Input: part model. Units: mm. Frame: model coordinates. A direction names the side the tool comes from. Coordinates: 2 decimals unless noted, no trailing zeros. Write each loop counter-clockwise with the first axis right and the second up, starting at its lowest first coordinate (ties: lowest second). Pieces come first, ordered by that corner, then holes. Notation, with made-up numbers: M 84,42 L 124,42 A21 cw 124,80 Z; hole C 18,70 d5. An arc over 180 degrees is marked long. Write each question's results on one line, items separated by ' | '. Start each with the question number.
1. Section query A-A, the plane y = 205. Output: boundary loops of the cut face in (x, z).
2. Pull-direction query (Y, two-part tool) for faces 3 (the flat face through (203.2, 154, 3)), 4 (the cylindrical face through (173.115, 253.638, 3.131)), 5 (the cylindrical face through (201.29, 1.81, 3.22)); classes: +Y half, -Y half, draft (parallel to the pull), parting line (faces both ways), or undercut.
3. Section query B-B, the plane x = 126.5. Output: boundary loops of the cut face in (y, z), and give its area (3 significant figures).
4. First-contact query: pin 1 (4.5 mm diameter, centred on x = 190.5, y = 241.3, fed in from -Z); pin 2 (1.5 mm diameter, centred on x = 167, z = 1.5, fed in from +Y); pin 3 (3 mm diameter, centred on y = 176.5, z = 2, fed in from -X); pin 4 (1.9 mm diameter, centred on x = 101, z = 3.5, fed in from +Y). Flat tips, straight axial feed; report the tip coordinate or a pass-through.
5. Set-up query: faces 1 (the flat face through (177.8, 138, 3)), 2 (the flat face through (95, 142, 0)). Return all of +Z, -Z, +X, -X, +Y, -Y with unobstructed straight access to the full face (end or side cutting, diameter ignored); none if empty.
6. Ray query, probe 1 along Y at (x, z) = (139.7, 5); probe 2 along Y at (x, z) = (38.1, 4.25); probe 3 along X at (y, z) = (133, 0.75). Return the intervals inside material, ascending.
```python
from build123d import *

# Parameters (mm, degrees)
BOSS_EXTRUDE1_DEPTH = 6.35
SKETCH2_R           = 2.4892
CUT_EXTRUDE1_DEPTH  = 7.35
FILLET1_R           = 6.35


with BuildPart() as part:
    # Sketch1 → Boss-Extrude1 (new body)
    with BuildSketch(Plane.XY):
        Polygon((0, 25.4), (177.8, 304.8), (203.2, 304.8), (203.2, 0), (0, 0), align=None)
    extrude(amount=BOSS_EXTRUDE1_DEPTH)

    # Sketch2 → Cut-Extrude1 (cut, through all)
    with BuildSketch(Plane.XY.offset(6.35)):
        with Locations((190.5, 12.7)):
            Circle(SKETCH2_R)
        with Locations((165.1, 12.7)):
            Circle(SKETCH2_R)
        with Locations((139.7, 12.7)):
            Circle(SKETCH2_R)
        with Locations((114.3, 12.7)):
            Circle(SKETCH2_R)
        with Locations((88.9, 12.7)):
            Circle(SKETCH2_R)
        with Locations((63.5, 12.7)):
            Circle(SKETCH2_R)
        with Locations((38.1, 12.7)):
            Circle(SKETCH2_R)
        with Locations((190.5, 38.1)):
            Circle(SKETCH2_R)
        with Locations((190.5, 63.5)):
            Circle(SKETCH2_R)
        with Locations((190.5, 88.9)):
            Circle(SKETCH2_R)
        with Locations((190.5, 114.3)):
            Circle(SKETCH2_R)
        with Locations((190.5, 139.7)):
            Circle(SKETCH2_R)
        with Locations((190.5, 165.1)):
            Circle(SKETCH2_R)
        with Locations((190.5, 190.5)):
            Circle(SKETCH2_R)
        with Locations((190.5, 215.9)):
            Circle(SKETCH2_R)
        with Locations((190.5, 241.3)):
            Circle(SKETCH2_R)
        with Locations((190.5, 266.7)):
            Circle(SKETCH2_R)
        with Locations((190.5, 292.1)):
            Circle(SKETCH2_R)
        with Locations((12.7, 12.7)):
            Circle(SKETCH2_R)
        Polygon((22.580146513, 25.4), (177.8, 25.4), (177.8, 269.316912623), align=None)
    extrude(amount=-CUT_EXTRUDE1_DEPTH, mode=Mode.SUBTRACT)

    # Fillet1
    fillet1_edges = [part.edges().sort_by_distance(p)[0] for p in [
        (22.580146513, 25.4, 3.175),
        (177.8, 269.316912623, 3.175),
        (177.8, 25.4, 3.175),
        (203.2, 0, 3.175),
        (0, 0, 3.175),
        (0, 25.4, 3.175),
        (177.8, 304.8, 3.175),
        (203.2, 304.8, 3.175),
    ]]
    fillet(fillet1_edges, radius=FILLET1_R)


solid = part.part
```
Answer:
1) outline: M 114.29,0 L 136.87,0 L 136.87,6.35 L 114.29,6.35 Z; M 177.8,0 L 203.2,0 L 203.2,6.35 L 177.8,6.35 Z
2) face 3: draft | face 4: undercut | face 5: -Y half
3) outline: M 0,0 L 25.4,0 L 25.4,6.35 L 0,6.35 Z; M 188.7,0 L 224.19,0 L 224.19,6.35 L 188.7,6.35 Z | area: 387 mm^2
4) pin 1: through | pin 2: y = 289.01 | pin 3: x = 95.2 | pin 4: y = 185.61
5) face 1: +Z, -Z | face 2: -Z, +X, -X, +Y, -Y
6) probe 1: 0 to 10.21, 15.19 to 25.4, 209.45 to 244.93 | probe 2: 0 to 10.21, 15.19 to 25.4, 49.79 to 85.27 | probe 3: 68.47 to 91.05, 177.8 to 203.2
